Autodesk Inventor part; units mm, degrees
ref_plane "YZ Plane" through (0, 0, 0) normal (1, 0, 0) x (0, 1, 0)
ref_plane "XZ Plane" through (0, 0, 0) normal (0, 1, 0) x (-1, 0, 0)
ref_plane "XY Plane" through (0, 0, 0) normal (0, 0, 1) x (1, 0, 0)
sketch "Sketch1" plane through (0, 0, 0) normal (0, 0, 1) x (1, 0, 0)
  circle A0 centre (0, 0) radius 29
  dimension "d1" = 58
extrude "Extrusion1" add sketch "Sketch1" along normal blind 2
sketch "Sketch3" plane through (0, 0, 2) normal (0, 0, 1) x (1, 0, 0)
  circle A0 centre (0, 0) radius 19
  dimension "d11" = 38
extrude "Extrusion2" add sketch "Sketch3" along normal blind 10
sketch "Sketch4" plane through (0, 0, 12) normal (0, 0, 1) x (1, 0, 0)
  point P0 (0, 0)
  point P1 (0, 0)
hole "Hole2" at (0, 0, 12) direction (0, 0, -1) diameter 33.5 depth 12 tip angle 118
properties part number "xiq_camera_holder"
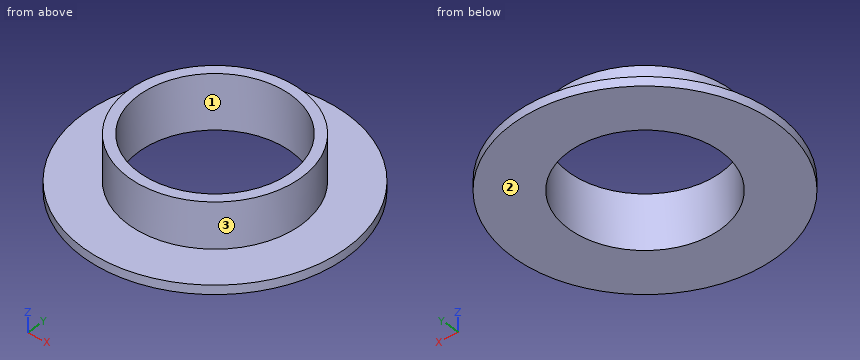
Source: CAD feature listing. Evaluate the final solid. Frame: model axes, mm. Face numbers are marked on the shaded views. Round coordinates to 2 decimals unless told otherwise and drop trailing zeros. Order: outer loops, then holes, each group sorted by start corner. A loop starts at its lowest first (then second) coordinate and runs counter-clockwise, first axis right, second up. Notation, with made-up numbers: (4, 82) -> (49, 82) arc R5 cw to (49, 86) -> close; hole circle Ø10 at (7, 40.25). An arc over 180 degrees is marked (long way). One line per item, written item: value. Start each with the question number.
Q1. Draft query along Y for the marked faces 1, 2 and 3. Return one class per face: pulls with the +Y half, pulls with the -Y half, needs draft (parallel to the pull), parting line crosses it, or undercut.
Q2. Pin query (flat end, axial travel): pin 1 (1 mm diameter, centred on y = -6, z = 8, fed in from +X); pin 2 (3 mm diameter, centred on x = 1, z = 5, fed in from +Y); pin 3 (1.5 mm diameter, centred on y = 14.5, z = 3, fed in from +X). Return the tip coordinate at first contact, or that it passes through.
Q3. Section query D-D (x = -23.5). Return the cut outline in (y, z).
Q4. Section query A-A (x = 0). Return the cut outline in (y, z).
Q5. Section query C-C (z = 4.5). Return the cut outline in (x, y), plus the area to 3 significant figures.
Q6. Material intervals for probe 1 along Y at (x, z) = (0, 9.5); probe 2 along Z at (x, y) = (-8.5, 18); probe 3 along X at (y, z) = (-11.5, 3.5), sorted ascending.
Findings below:
1. face 1: undercut
1. face 2: needs draft
1. face 3: parting line crosses it
2. pin 1: x = 18.19
2. pin 2: y = 19
2. pin 3: x = 13.11
3. outline: (-16.99, 0) -> (16.99, 0) -> (16.99, 2) -> (-16.99, 2) -> close
4. outline: (-29, 0) -> (-16.75, 0) -> (-16.75, 12) -> (-19, 12) -> (-19, 2) -> (-29, 2) -> close; (16.75, 0) -> (29, 0) -> (29, 2) -> (19, 2) -> (19, 12) -> (16.75, 12) -> close
5. outline: circle Ø38 at (0, 0); hole circle Ø33.5 at (0, 0)
5. area: 253 mm²
6. probe 1: -19 to -16.75, 16.75 to 19
6. probe 2: 0 to 2
6. probe 3: -15.12 to -12.18, 12.18 to 15.12
